```python
from build123d import *

# Parameters (mm, degrees)
CROQUIS2_W                   = 275.5
CROQUIS2_H                   = 43
CROQUIS2_R                   = 4
CROQUIS2_R_2                 = 4.5
CROQUIS2_R_3                 = 12
SALIENTE_EXTRUIR1_DEPTH      = 3
REDONDEO1_R                  = 5
TALADRO_DE_MARGEN_PARA_M41_D = 4.5
TALADRO_DE_MARGEN_PARA_M31_D = 3.4
TALADRO_DE_MARGEN_PARA_M42_D = 4.5


with BuildPart() as part:
    # Croquis2 → Saliente-Extruir1 (new, symmetric)
    with BuildSketch(Plane(origin=(0, 0, 0), x_dir=(0, 0, -1), z_dir=(1, 0, 0))):
        with Locations((-20.25, 0)):
            Rectangle(CROQUIS2_W, CROQUIS2_H)
        with Locations((-100, 0)):
            Circle(CROQUIS2_R, mode=Mode.SUBTRACT)
        with Locations((100, 0)):
            Circle(CROQUIS2_R_2, mode=Mode.SUBTRACT)
        with Locations((-135, 0)):
            Circle(CROQUIS2_R_3, mode=Mode.SUBTRACT)
    extrude(amount=SALIENTE_EXTRUIR1_DEPTH, both=True)

    # Redondeo1
    redondeo1_edges = [part.edges().sort_by_distance(p)[0] for p in [
        (0, 21.5, 158),
        (0, 21.5, -117.5),
        (0, -21.5, -117.5),
        (0, -21.5, 158),
    ]]
    fillet(redondeo1_edges, radius=REDONDEO1_R)

    # Taladro de margen para M41 (through all)
    with Locations(Plane(origin=(3, 0, 0), x_dir=(0, 0, -1), z_dir=(1, 0, 0))):
        with Locations((112.5, 12.5), (112.5, -12.5), (87.5, -12.5), (87.5, 12.5)):
            Hole(TALADRO_DE_MARGEN_PARA_M41_D / 2)

    # Taladro de margen para M31 (through all)
    with Locations(Plane.ZY.offset(3)):
        with Locations((150.5, 15.5), (119.5, 15.5), (119.5, -15.5), (150.5, -15.5)):
            Hole(TALADRO_DE_MARGEN_PARA_M31_D / 2)

    # Taladro de margen para M42 (through all)
    with Locations(Plane.ZY.offset(3)):
        with Locations((-40, 0), (40, 0)):
            Hole(TALADRO_DE_MARGEN_PARA_M42_D / 2)


solid = part.part
```
Work out the finished part from the listing and answer in its coordinate system (mm). Give positions to 0.01 mm unless a question says otherwise; leave off trailing zeros. Order: outer loops, then holes, each group sorted by start corner. A loop starts at its lowest first (then second) coordinate and runs counter-clockwise, first axis right, second up. Notation, with made-up numbers: (-26.5, -13) -> (18.5, -13) arc R24 cw to (18.5, 17) -> close; hole circle Ø4 at (-19, 27). An arc over 180 degrees is marked (long way). Answer as CSV lines item,"result". Start each with the question number.
(1) Consider line 1 along Y through (x, z) = (-1.65, -87.5); line 2 along Y through (x, z) = (-1.2, 100); line 3 along Y through (x, z) = (-1.05, 135). Determine where each line is inside the solid, lowest interval first.
(2) Section B-B, the plane z = 135 is taken. Write down the section's boundary in (x, y).
(3) Section C-C, the plane x = 0.65 is taken. Give the number of separate pieces and of enclosed holes in the cut face, plus the area to 3 significant figures.
(4) Section A-A, the plane y = 0 is taken. Write down the section's boundary in (x, z).
(5) For a pull along Z with two mould halves and no side action, classify faces 1 (the cylindrical face through (-0.042, 13.176, -110.354)), 2 (the cylindrical face through (-0.04, 20, -116.07)), 3 (the cylindrical face through (-0.04, 20, 156.57)) as released by +Z, released by -Z, zero draft, split by the parting line, or undercut.
(6) This flat-tipped pin is pushed along its axis until it touches: pin 1 Ø3.5 at (y, z) = (12.5, -112.5) entering from -X. Where does it stop, or does it pass through?
(7) Section D-D, the plane z = -87.5 is taken. Write down the section's boundary in (x, y), plus the area to 3 significant figures.
Entries:
1,line 1,"-21.5 to -14.75, -10.25 to 10.25, 14.75 to 21.5"
1,line 2,"-21.5 to -4, 4 to 21.5"
1,line 3,"-21.5 to -12, 12 to 21.5"
2,outline,"(-3, -21.5) -> (3, -21.5) -> (3, -12) -> (-3, -12) -> close; (-3, 12) -> (3, 12) -> (3, 21.5) -> (-3, 21.5) -> close"
3,separate pieces,"1"
3,enclosed holes,"13"
3,area,"11,100 mm²"
4,outline,"(-3, -117.5) -> (3, -117.5) -> (3, -104.5) -> (-3, -104.5) -> close; (-3, -95.5) -> (3, -95.5) -> (3, -42.25) -> (-3, -42.25) -> close; (-3, -37.75) -> (3, -37.75) -> (3, 37.75) -> (-3, 37.75) -> close; (-3, 42.25) -> (3, 42.25) -> (3, 96) -> (-3, 96) -> close; (-3, 104) -> (3, 104) -> (3, 123) -> (-3, 123) -> close; (-3, 147) -> (3, 147) -> (3, 158) -> (-3, 158) -> close"
5,face 1,"undercut"
5,face 2,"released by -Z"
5,face 3,"released by +Z"
6,pin 1,"through"
7,outline,"(-3, -21.5) -> (3, -21.5) -> (3, -14.75) -> (-3, -14.75) -> close; (-3, -10.25) -> (3, -10.25) -> (3, 10.25) -> (-3, 10.25) -> close; (-3, 14.75) -> (3, 14.75) -> (3, 21.5) -> (-3, 21.5) -> close"
7,area,"204 mm²"
